```python
from build123d import *

# Parameters (mm, degrees)
F1_DEPTH = 10
F2_DEPTH = 20
F3_R     = 1


with BuildPart() as f1:
    # F0 (on Top) → F1 (new body)
    with BuildSketch(Plane.XY):
        Polygon((4.571693, 2.589007), (0.0437, 5.253706), (-4.527993, 2.664698), (-4.571693, -2.589007), (-0.0437, -5.253706), (4.527993, -2.664698), align=None)
    extrude(amount=F1_DEPTH)

    # F0 (on Top) → F2 (join)
    with BuildSketch(Plane.XY):
        Polygon((6.589365, 3.712885), (0.07923, 7.563), (-6.510135, 3.850115), (-6.589365, -3.712885), (-0.07923, -7.563), (6.510135, -3.850115), align=None)
        Polygon((-4.527993, 2.664698), (0.0437, 5.253706), (4.571693, 2.589007), (4.527993, -2.664698), (-0.0437, -5.253706), (-4.571693, -2.589007), align=None, mode=Mode.SUBTRACT)
    extrude(amount=F2_DEPTH)

    # F3
    f3_edges = [f1.edges().sort_by_distance(p)[0] for p in [
        (3.215452, -5.706557, 0),
        (-3.334297, -5.637942, 0),
        (-6.54975, 0.068615, 0),
        (-3.215452, 5.706557, 0),
        (3.334297, 5.637942, 0),
        (6.54975, -0.068615, 0),
    ]]
    fillet(f3_edges, radius=F3_R)


solid = f1.part
```
Here's how the part is built. I have some questions about the finished solid (model axes, mm). A direction names the side the tool comes from. Coordinates: 2 decimals unless noted, no trailing zeros. Order: outer loops, then holes, each group sorted by start corner. A loop starts at its lowest first (then second) coordinate and runs counter-clockwise, first axis right, second up.
Item 1: I'm going to push flat-ended pins straight in: pin 1 Ø6 at (y, z) = (-5, 9.5) entering from +X; pin 2 Ø3 at (x, z) = (-3.5, 6.5) entering from -Y; pin 3 Ø5 at (x, z) = (-2.5, 14) entering from +Y. Where does each tip first touch, or does it pass through?
Response values:
pin 1: stops at x = 6.53
pin 2: stops at y = -6.43
pin 3: stops at y = 7.52
Item 2: Thinking about a two-plate mould opening in X: for faces 4 (the face through (3.4, 5.6, 10.4)), 5 (the face through (0, 0, 0)), 6 (the face through (2.274, -3.941, 14.93)), which applies, pulls with the +X half, pulls with the -X half, needs draft (parallel to the pull), parting line crosses it, or undercut?
Response values:
face 4: pulls with the +X half
face 5: needs draft
face 6: undercut
Item 3: If we section it at A-A, the plane z = 13.75: List the corners of the cut face in (x, y) for me, then the cut area to 3 significant figures.
Response values:
outline: (-6.59, -3.71) - (-0.08, -7.56) - (6.51, -3.85) - (6.59, 3.71) - (0.08, 7.56) - (-6.51, 3.85) - close; hole (-4.57, -2.59) - (-0.04, -5.25) - (4.53, -2.66) - (4.57, 2.59) - (0.04, 5.25) - (-4.53, 2.66) - close
area: 76.9 mm2
Item 4: Which directions (+Z, -Z, +X, -X, +Y, -Y) give clear straight access to the entire face, cutting with the end or side of a thin tool? Please do faces 1 (the face through (6.265, -0.013, 0.301)), 2 (the face through (0, 0, 10)), 3 (the face through (-6.25, 0.013, 0.285)).
Response values:
face 1: -Z, +X, -Y
face 2: +Z
face 3: -Z, -X, +Y
Item 5: If we section it at B-B, the plane z = 7: List the corners of the cut face in (x, y) for me.
Response values:
outline: (-6.59, -3.71) - (-0.08, -7.56) - (6.51, -3.85) - (6.59, 3.71) - (0.08, 7.56) - (-6.51, 3.85) - close
Item 6: I need wall thicknesses on probe 1 along Z at (x, y) = (2.5, -3); probe 2 along X at (y, z) = (-3, 10.5); probe 3 along X at (y, z) = (1.75, 10.25). Which ranges of each line are inside material? Lowest first, please.
Response values:
probe 1: z = 0 to 10
probe 2: x = -6.58 to -3.87, 3.94 to 6.52
probe 3: x = -6.53 to -4.54, 4.56 to 6.57
